Autodesk Inventor part; units mm, degrees
ref_plane "YZ Plane" through (0, 0, 0) normal (1, 0, 0) x (0, 1, 0)
ref_plane "XZ Plane" through (0, 0, 0) normal (0, 1, 0) x (-1, 0, 0)
ref_plane "XY Plane" through (0, 0, 0) normal (0, 0, 1) x (1, 0, 0)
sketch "Sketch1" plane through (0, 0, 0) normal (1, 0, 0) x (0, 1, 0)
  line L0 (0, 25.4) -> (0, 0)
  line L1 (0, 0) -> (25.4, 0)
  line L2 (25.4, 0) -> (25.4, 6.35)
  line L3 (25.4, 6.35) -> (9.525, 6.35)
  line L4 (6.35, 9.525) -> (6.35, 25.4)
  line L5 (6.35, 25.4) -> (0, 25.4)
  arc A0 (6.35, 9.525) -> (9.525, 6.35) centre (9.525, 9.525) ccw
  dimension "d0" = 3.175
  dimension "d1" = 25.4
  dimension "d2" = 6.35
extrude "Extrusion1" add sketch "Sketch1" along normal blind 38.1
sketch "Sketch2" plane through (0, 0, 0) normal (0, 0, -1) x (-1, 0, 0)
  line L0 (0, 6.35) -> (-38.1, 6.35) construction
  line L1 (0, 25.4) -> (-38.1, 25.4) construction
  circle A0 centre (-28.575, 15.875) radius 1.905
  line L2 (-28.575, 25.4) -> (-28.575, 6.35) construction
  line L3 (-19.05, 6.35) -> (-19.05, 25.4) construction
  line L4 (-9.525, 25.4) -> (-9.525, 6.35) construction
  circle A1 centre (-9.525, 15.875) radius 1.905
  point P0 (0, 0)
  dimension "d5" = 3.81
  dimension "d11" = 19.05
extrude "Extrusion2" cut sketch "Sketch2" against normal through all
sketch "Sketch3" plane through (0, 0, 0) normal (0, -1, 0) x (1, 0, 0)
  line L0 (0, 6.35) -> (38.1, 6.35) construction
  line L1 (26.67, 6.35) -> (30.48, 6.35) construction
  line L2 (0, 25.4) -> (38.1, 25.4) construction
  circle A0 centre (19.05, 15.875) radius 1.905
  line L3 (0, 25.4) -> (38.1, 25.4) construction
  line L4 (19.05, 25.4) -> (19.05, 6.35) construction
  point P0 (0, 0)
  point P1 (19.05, 15.875)
  dimension "d8" = 3.81
extrude "Extrusion3" cut sketch "Sketch3" against normal through all
properties part number "Tension Angle"
Model file for the job. Use its own axes, mm. A direction names the side the tool comes from. Coordinates: 2 decimals unless noted, no trailing zeros. Loops run counter-clockwise (first coordinate to the right, second up) from the corner with the lowest first, then second, coordinate; pieces in that order, holes last. Notation, with made-up numbers: M -8,74 L 23,74 A27 cw 23,96 Z; hole C -38,3.25 d11. An arc over 180 degrees is marked long. Use CSV: the item, a comma, the result in double quotes. Start each with the question number.
1. Band-saw the part on D-D, the plane y = 7.5. List the corners of the cut face in (x, z).
2. Flat gauge pins, fed straight in: pin 1 (3 mm diameter, centred on x = 30, z = 20, fed in from -Y); pin 2 (3 mm diameter, centred on x = 31.5, y = 12, fed in from +Z); pin 3 (3 mm diameter, centred on x = 28.575, y = 15.875, fed in from +Z); pin 4 (5 mm diameter, centred on x = 24.5, z = 19, fed in from +Y). Where does each tip first touch, or does it go through?
3. Band-saw the part on C-C, the plane z = 4. List the corners of the cut face in (x, y) (3 decimals), then the cut area to 3 significant figures.
4. Tool access for faces 1 (the flat face through (19, 18, 6.35)), 2 (the cylindrical face through (8.646, 14.185, 3.131)): list every direction of +Z, -Z, +X, -X, +Y, -Y with a clear straight run to the whole face (end or side of a thin tool).
5. Probe probe 1 along Z at (x, y) = (19.05, 4.5); probe 2 along Z at (x, y) = (36, 11.25). List the from-to ranges inside material, lowest first. Write a range as [from, to].
6. Band-saw the part on B-B, the plane x = 12.5. List the corners of the cut face in (y, z) (3 decimals), then the cut area to 3 significant figures.
7. Band-saw the part on A-A, the plane x = 19.05. List the corners of the cut face in (y, z) (3 decimals), then the cut area to 3 significant figures.
8. Two-plate mould, pull along Y, no slides. Class faces 3 (the flat face through (19, 6.35, 19)), 4 (the cylindrical face through (17.538, 3.131, 14.716)), 5 (the cylindrical face through (26.815, 15.145, 3.131)): pulls with the +Y half, pulls with the -Y half, needs draft (parallel to the pull), parting line crosses it, or undercut.
Entries:
1,outline,"M 0,0 L 38.1,0 L 38.1,7.08 L 0,7.08 Z"
2,pin 1,"stops at y = 0"
2,pin 2,"stops at z = 6.35"
2,pin 3,"passes through"
2,pin 4,"stops at y = 6.35"
3,outline,"M 0,0 L 38.1,0 L 38.1,25.4 L 0,25.4 Z; hole C 9.525,15.875 d3.81; hole C 28.575,15.875 d3.81"
3,area,"945 mm2"
4,face 1,"+Z, +X, -X, +Y"
4,face 2,"+Z, -Z"
5,probe 1,"z = [0, 13.97], [17.78, 25.4]"
5,probe 2,"z = [0, 6.35]"
6,outline,"M 0,0 L 25.4,0 L 25.4,6.35 L 9.525,6.35 A3.175 cw 6.35,9.525 L 6.35,25.4 L 0,25.4 Z"
6,area,"284 mm2"
7,outline,"M 0,0 L 25.4,0 L 25.4,6.35 L 9.525,6.35 A3.175 cw 6.35,9.525 L 6.35,13.97 L 0,13.97 Z; M 0,17.78 L 6.35,17.78 L 6.35,25.4 L 0,25.4 Z"
7,area,"260 mm2"
8,face 3,"pulls with the +Y half"
8,face 4,"needs draft"
8,face 5,"undercut"
